Check sheet for the drawn part. Datum: minimum x, y, z corner. Units: mm. A direction names the side the tool comes from. Coordinates: 2 decimals unless noted, no trailing zeros. Loops run counter-clockwise (first coordinate to the right, second up) from the corner with the lowest first, then second, coordinate; pieces in that order, holes last.
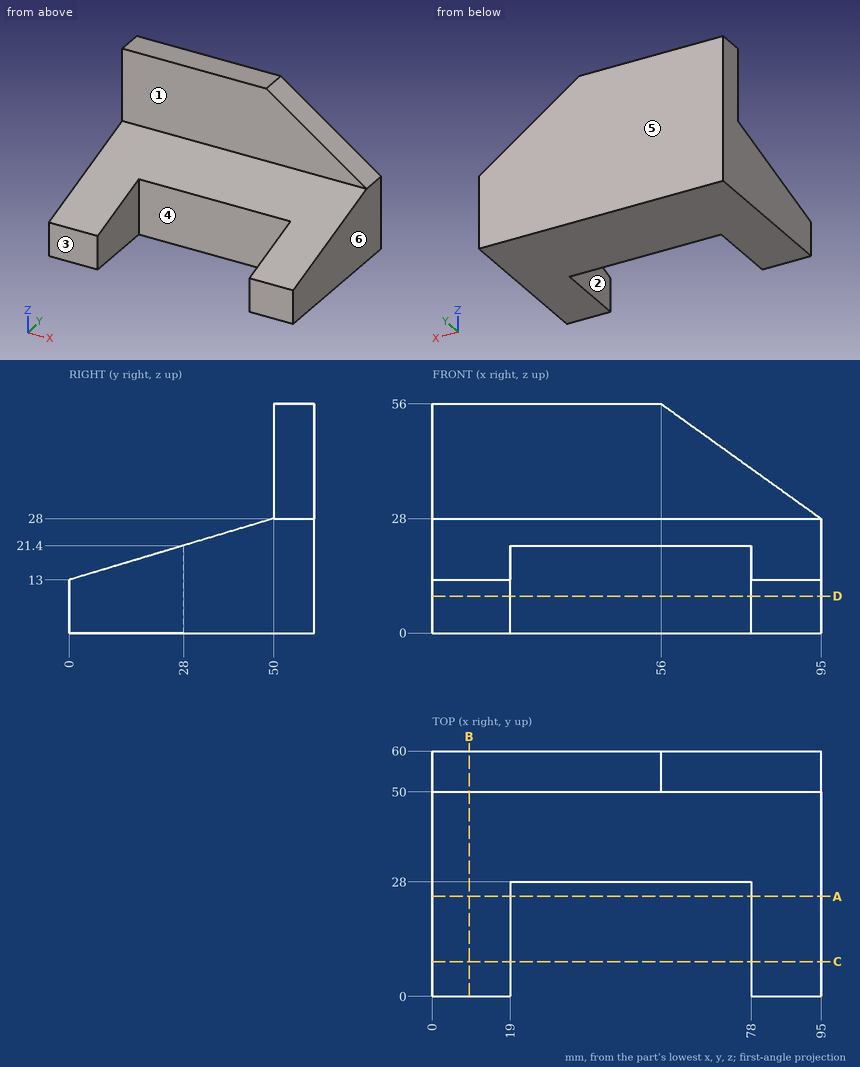
1) Section check A-A on y = 24.5. Enter the section's corners in (x, z).
Answer sheet:
outline: (0, 0) - (19, 0) - (19, 20.35) - (0, 20.35) - close; (78, 0) - (95, 0) - (95, 20.35) - (78, 20.35) - close
2) Set-up check for the marked faces 1, 2 and 3: record each of +Z, -Z, +X, -X, +Y, -Y from which the full face is reachable in a straight line by a thin tool's end or side.
Answer sheet:
face 1: +Z, +X, -X, -Y
face 2: +Z, -Z, -Y
face 3: +Z, -Z, +X, -X, -Y
3) Section check B-B on x = 9. Enter the section's corners in (y, z), plus the area to 4 significant figures.
Answer sheet:
outline: (0, 0) - (60, 0) - (60, 56) - (50, 56) - (50, 28) - (0, 13) - close
area: 1,585 mm2
4) Mould release check, pull along X, two halves, no side actions. Record for the marked faces 4, 5 and 6: +X half, -X half, draft (parallel to the pull), parting line (faces both ways), or undercut.
Answer sheet:
face 4: undercut
face 5: draft
face 6: +X half
5) Depth check by flat-ended pin: pin 1 (12 mm diameter, centred on x = 61, z = 15, fed in from -Y); pin 2 (1.5 mm diameter, centred on x = 78, y = 38, fed in from +Z) (3 decimals). Enter the tip coordinate at first touch or a pass-through.
Answer sheet:
pin 1: stops at y = 28
pin 2: stops at z = 24.625
6) Scan lines: line 1 (X direction, y = 18.5, z = 6.5); line 2 (Y direction, x = 17, z = 47.5); line 3 (Y direction, x = 44.5, z = 15). Record each from-to range of solid material in increasing order.
Answer sheet:
line 1: x = 0 to 19, 78 to 95
line 2: y = 50 to 60
line 3: y = 28 to 60
7) Section check D-D on z = 9. Enter the section's corners in (x, y).
Answer sheet:
outline: (0, 0) - (19, 0) - (19, 28) - (78, 28) - (78, 0) - (95, 0) - (95, 60) - (0, 60) - close
8) Section check C-C on y = 8.5. Enter the section's corners in (x, z), plus the area to 3 significant figures.
Answer sheet:
outline: (0, 0) - (19, 0) - (19, 15.55) - (0, 15.55) - close; (78, 0) - (95, 0) - (95, 15.55) - (78, 15.55) - close
area: 560 mm2
